Work out the finished part from the listing and answer in its coordinate system (mm). A direction names the side the tool comes from. Round coordinates to 2 decimals unless told otherwise and drop trailing zeros. Loops run counter-clockwise (first coordinate to the right, second up) from the corner with the lowest first, then second, coordinate; pieces in that order, holes last.
```python
from build123d import *

# Parameters (mm, degrees)
SKETCH1_W          = 35
SKETCH1_H          = 33
BASE_FLANGE1_DEPTH = 3
EDGE_FLANGE1_DEPTH = 35


# Sheet-metal steps are written as plain solids
with BuildPart() as part:
    # Sketch1 → Base-Flange1 (new body)
    with BuildSketch(Plane(origin=(0, 0, 0), x_dir=(0, 0, -1), z_dir=(1, 0, 0))):
        with Locations((-1713.733243968, 358.835120643)):
            Rectangle(SKETCH1_W, SKETCH1_H)
    extrude(amount=-BASE_FLANGE1_DEPTH)

    # Edge-Flange1 section (across the edge) → Edge-Flange1 (add)
    with BuildSketch(Plane(origin=(0, 378.335120643, 1696.233243968), x_dir=(0, -1, 0), z_dir=(0, 0, 1))):
        with BuildLine():
            Line((-3, 3), (-3, 47))
            Line((-3, 47), (0, 47))
            Line((0, 47), (0, 3))
            ThreePointArc((0, 3), (0.878679656, 0.878679656), (3, 0))
            Line((3, 0), (3, -3))
            ThreePointArc((3, -3), (-1.242640687, -1.242640687), (-3, 3))
        make_face()
    extrude(amount=EDGE_FLANGE1_DEPTH)


solid = part.part
```
1. Find section C-C (x = 19.5). Write down the section's boundary in (y, z).
Answer key:
outline: (378.34, 1696.23) - (381.34, 1696.23) - (381.34, 1731.23) - (378.34, 1731.23) - close
2. Find section B-B (y = 352). Write down the section's boundary in (x, z), then the cut area to 3 significant figures.
Answer key:
outline: (-3, 1696.23) - (0, 1696.23) - (0, 1731.23) - (-3, 1731.23) - close
area: 105 mm2
3. Given pin 1 (2 mm diameter, centred on y = 358.5, z = 1701, fed in from +X); pin 2 (10 mm diameter, centred on x = 21.5, z = 1704, fed in from -Y), each flat-ended and moving along its own axis, determine where each tip first touches the part or whether it passes through.
Answer key:
pin 1: stops at x = 0
pin 2: stops at y = 378.34
4. Consider probe 1 along X at (y, z) = (364.5, 1716.5); probe 2 along Y at (x, z) = (15, 1726); probe 3 along Y at (x, z) = (0.5, 1709). Determine where each line is inside the solid, lowest interval first.
Answer key:
probe 1: x = -3 to 0
probe 2: y = 378.34 to 381.34
probe 3: y = 376.99 to 380.79
5. Which of the six approach directions +Z, -Z, +X, -X, +Y, -Y give full straight-line access (tool end or side, diameter ignored) to faces 1 (the face through (25, 381.335, 1713)), 2 (the face through (25, 378.335, 1713))?
Answer key:
face 1: +Z, -Z, +X, -X, +Y
face 2: +Z, -Z, +X, -Y
6. Find section A-A (z = 1714). Write down the section's boundary in (x, y), then the cut area to 3 significant figures.
Answer key:
outline: (-3, 342.34) - (0, 342.34) - (0, 375.34) arc R3 cw to (3, 378.34) - (47, 378.34) - (47, 381.34) - (3, 381.34) arc R6 ccw to (-3, 375.34) - close
area: 252 mm2
